Here's how the part is built. I have some questions about the finished solid (model axes, mm). Face numbers are marked on the shaded views. A direction names the side the tool comes from. Round coordinates to 2 decimals unless told otherwise and drop trailing zeros. Write each loop counter-clockwise with the first axis right and the second up, starting at its lowest first coordinate (ties: lowest second). Pieces come first, ordered by that corner, then holes. Notation, with made-up numbers: (41.5, -16.5) -> (85.5, -16.5) arc R12 ccw to (85.5, -8.5) -> close; hole circle Ø8 at (-39.5, 54.25). An arc over 180 degrees is marked (long way). Put each result on its own line as item: value. Start each with the question number.
1) I want a section at B-B, the plane x = 7.5. List the corners of the cut face in (y, z) for me.
2) I want a section at A-A, the plane z = 0. List the corners of the cut face in (x, y) for me, then the cut area to 3 significant figures.
3) Which directions (+Z, -Z, +X, -X, +Y, -Y) give clear straight access to the entire face, cutting with the end or side of a thin tool? Please do the marked faces 1 and 2.
4) If I drill on line 1 along Z through (x, y) = (3, -0.5); line 2 along X through (y, z) = (-0.8, 1.5); line 3 along Y through (x, z) = (9.5, 0.9), over which ranges is the centre line in solid material (lowest first)? Write a range as [from, to].
5) Will these pins go through, and if not, where does the flat tip stop? P1, Ø1.5, axis at x = 7, z = 0, coming from the +Y side; P2, Ø2, axis at x = 1.5, z = -1.5, coming from the +Y side.
from build123d import *

# Parameters (mm, degrees)
CUT_EXTRUDE1_DEPTH = 0.8


with BuildPart() as part:
    # Sketch2 → Revolve1 (revolve)
    with BuildSketch(Plane.XY):
        with BuildLine():
            Line((0, 0), (0, 1.8))
            ThreePointArc((0, 1.8), (0.058578644, 1.941421356), (0.2, 2))
            Line((0.2, 2), (1.8, 2))
            ThreePointArc((1.8, 2), (1.941421356, 1.941421356), (2, 1.8))
            Line((2, 1.8), (2, 1))
            Line((2, 1), (11.75, 1))
            Line((11.75, 1), (12, 0.75))
            Line((12, 0.75), (12, 0))
            Line((12, 0), (0, 0))
        make_face()
    revolve(axis=Axis((-2.281841559, 0, 0), (1, 0, 0)))

    # Sketch3 → Cut-Extrude1 (cut)
    with BuildSketch(Plane.ZY):
        Polygon((0.433012702, -0.75), (0.866025404, 0), (0.433012702, 0.75), (-0.433012702, 0.75), (-0.866025404, 0), (-0.433012702, -0.75), align=None)
    extrude(amount=-CUT_EXTRUDE1_DEPTH, mode=Mode.SUBTRACT)


solid = part.part
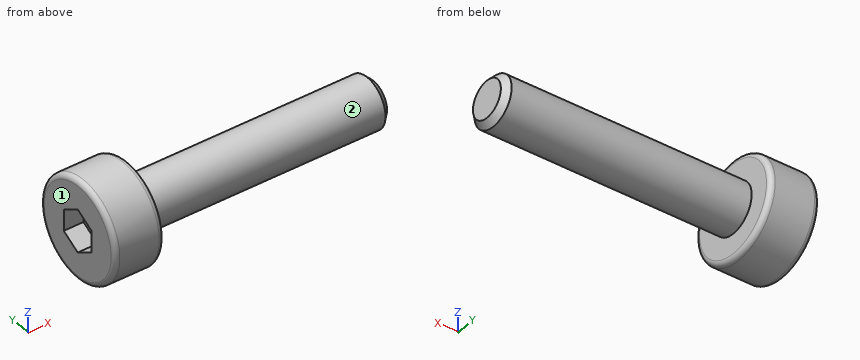
Findings:
1. outline: circle Ø2 at (0, 0)
2. outline: (0, -1.8) arc R0.2 ccw to (0.2, -2) -> (1.8, -2) arc R0.2 ccw to (2, -1.8) -> (2, -1) -> (11.75, -1) -> (12, -0.75) -> (12, 0.75) -> (11.75, 1) -> (2, 1) -> (2, 1.8) arc R0.2 ccw to (1.8, 2) -> (0.2, 2) arc R0.2 ccw to (0, 1.8) -> (0, 0.75) -> (0.8, 0.75) -> (0.8, -0.75) -> (0, -0.75) -> close
2. area: 26.7 mm2
3. face 1: +Z, -Z, -X, +Y, -Y
3. face 2: +X
4. line 1: z = [-0.87, 0.87]
4. line 2: x = [0, 2]
4. line 3: y = [-0.44, 0.44]
5. P1: stops at y = 1
5. P2: stops at y = 1.94
